from build123d import *

# Parameters (mm, degrees)
SKETCH1_R                  = 2.5
BOSS_EXTRUDE1_DEPTH        = 95
CUT_EXTRUDE1_DEPTH         = 96.065766709
CUT_EXTRUDE1_DEPTH_BACK    = 96.065766709
SKETCH2_R                  = 1.5
CHAMFER1_SIZE              = 0.5
M3X0_5_TAPPED_HOLE1_REACH  = 97.066
M3X0_5_TAPPED_HOLE1_BORE_R = 1.25
CUT_EXTRUDE2_DEPTH         = 96.065766714
CUT_EXTRUDE2_DEPTH_BACK    = 96.065766714
SKETCH6_W                  = 16
SKETCH6_H                  = 0.5
M3X0_5_TAPPED_HOLE2_D      = 2.5


with BuildPart() as part:
    # Sketch1 → Boss-Extrude1 (new body)
    with BuildSketch(Plane.XY):
        Circle(SKETCH1_R)
    extrude(amount=BOSS_EXTRUDE1_DEPTH)

    # Sketch2 → Cut-Extrude1 (cut, two sides: drawn at the far end of the back side and taken through both)
    with BuildSketch(Plane(origin=(0, 0, 0), x_dir=(1, 0, 0), z_dir=(0, 1, 0)).offset(-CUT_EXTRUDE1_DEPTH_BACK)):
        with Locations(Location((0, -4, 0), (0, 0, 270))):
            Circle(SKETCH2_R)
    extrude(amount=CUT_EXTRUDE1_DEPTH + CUT_EXTRUDE1_DEPTH_BACK, mode=Mode.SUBTRACT)

    # Chamfer1
    chamfer1_edges = [part.edges().sort_by_distance(p)[0] for p in [
        (-2.5, 0, 0),
        (-2.5, 0, 95),
    ]]
    chamfer(chamfer1_edges, length=CHAMFER1_SIZE)

    # M3x0.5 Tapped Hole1 bore → M3x0.5 Tapped Hole1 (cut, up to next)
    with BuildSketch(Plane(origin=(0, 0, 0), x_dir=(-1, 0, 0), z_dir=(0, 0, -1)), mode=Mode.PRIVATE) as m3x0_5_tapped_hole1_sk1:
        Circle(M3X0_5_TAPPED_HOLE1_BORE_R)
    m3x0_5_tapped_hole1_tool1 = extrude(m3x0_5_tapped_hole1_sk1.sketch, amount=-M3X0_5_TAPPED_HOLE1_REACH, mode=Mode.PRIVATE) & part.part
    add(m3x0_5_tapped_hole1_tool1.solids().sort_by_distance((0, 0, 0))[0], mode=Mode.SUBTRACT)

    # Sketch6 → Cut-Extrude2 (cut, two sides: drawn at the far end of the back side and taken through both)
    with BuildSketch(Plane(origin=(0, 0, 0), x_dir=(0, 0, -1), z_dir=(1, 0, 0)).offset(-CUT_EXTRUDE2_DEPTH_BACK)):
        with Locations((-83, 2.25)):
            Rectangle(SKETCH6_W, SKETCH6_H)
    extrude(amount=CUT_EXTRUDE2_DEPTH + CUT_EXTRUDE2_DEPTH_BACK, mode=Mode.SUBTRACT)

    # M3x0.5 Tapped Hole2 (through all)
    with Locations(Plane(origin=(0, 3, 0), x_dir=(1, 0, 0), z_dir=(0, 1, 0))):
        with Locations((0, -42.3)):
            Hole(M3X0_5_TAPPED_HOLE2_D / 2)


solid = part.part
Here's how the part is built. I have some questions about the finished solid (model axes, mm). Coordinates: 2 decimals unless noted, no trailing zeros. Loops run counter-clockwise (first coordinate to the right, second up) from the corner with the lowest first, then second, coordinate; pieces in that order, holes last. Notation, with made-up numbers: (73.25, -19) -> (125.25, -19) arc R28 cw to (125.25, 18) -> close; hole circle Ø7 at (-37, 40.25). An arc over 180 degrees is marked (long way). Use one line per item in the form item = value. Start each with the question number.
(1) We'd pull the mould along Z, two halves only. Please class faces 1 (the face through (-0.672, 1.054, 1.563)), 2 (the face through (-1.155, -0.035, 42.779)), 3 (the face through (0, 0, 95)), 4 (the face through (0, 2, 83)): pulls with the +Z half, pulls with the -Z half, needs draft (parallel to the pull), parting line crosses it, or undercut.
(2) If we section it at A-A (x = 0): Please give me the cut outline in (y, z).
(3) If we section it at C-C (z = 4): Please give me the cut outline in (x, y).
(4) Please list where these lines run through material, in increasing order: line 1 along Z through (x, y) = (-0.15, 1.55); line 2 along Z through (x, y) = (1.1, 1.05); line 3 along Z through (x, y) = (-0.85, 2.15).
(5) Will these pins go through, and if not, where does the flat tip stop? pin 1 (2 mm diameter, centred on x = 0, z = 42.3, fed in from +Y); pin 2 (0.6 mm diameter, centred on x = 0.5, y = 2.5, fed in from +Z); pin 3 (1.5 mm diameter, centred on x = 1, z = 50, fed in from +Y); pin 4 (1.5 mm diameter, centred on x = 0.5, z = 85.5, fed in from +Y).
(6) If we section it at B-B (y = 0): Please give me the cut outline in (x, z), then the cut area to 3 significant figures.
(7) If we section it at D-D (z = 82.5): Please give me the cut outline in (x, y), then the cut area to 3 significant figures.
Verdict:
q1.face_1 = needs draft
q1.face_2 = undercut
q1.face_3 = pulls with the +Z half
q1.face_4 = undercut
q2.outline = (-2.5, 0.5) -> (-2, 0) -> (-1.25, 0) -> (-1.25, 2.5) -> (-2.5, 2.5) -> close; (-2.5, 5.5) -> (2.5, 5.5) -> (2.5, 41.05) -> (-2.5, 41.05) -> close; (-2.5, 43.55) -> (2.5, 43.55) -> (2.5, 75) -> (2, 75) -> (2, 91) -> (2.5, 91) -> (2.5, 94.5) -> (2, 95) -> (-2, 95) -> (-2.5, 94.5) -> close; (1.25, 0) -> (2, 0) -> (2.5, 0.5) -> (2.5, 2.5) -> (1.25, 2.5) -> close
q3.outline = (-1.5, -2) -> (-1.5, 2) arc R2.5 ccw to start; (1.5, -2) arc R2.5 ccw to (1.5, 2) -> close
q4.line_1 = 0 to 2.51, 5.49 to 41.06, 43.54 to 95
q4.line_2 = 0 to 2.98, 5.02 to 41.71, 42.89 to 95
q4.line_3 = 0.31 to 2.76, 5.24 to 41.38, 43.22 to 75, 91 to 94.69
q5.pin_1 = through
q5.pin_2 = 94.75
q5.pin_3 = 2.49
q5.pin_4 = 2
q6.outline = (-2.5, 0.5) -> (-2, 0) -> (-1.25, 0) -> (-1.25, 3.17) arc R1.5 cw (long way) to (1.25, 3.17) -> (1.25, 0) -> (2, 0) -> (2.5, 0.5) -> (2.5, 94.5) -> (2, 95) -> (-2, 95) -> (-2.5, 94.5) -> close; hole circle Ø2.5 at (0, 42.3)
q6.area = 456 mm²
q7.outline = (-1.5, 2) arc R2.5 ccw (long way) to (1.5, 2) -> close
q7.area = 18.6 mm²
